The model under review builds one solid part; all positions refer to its coordinate system, in mm. Face numbers are marked on the shaded views. A direction names the side the tool comes from. Give positions to 0.01 mm unless a question says otherwise; leave off trailing zeros. Order: outer loops, then holes, each group sorted by start corner. A loop starts at its lowest first (then second) coordinate and runs counter-clockwise, first axis right, second up. Notation, with made-up numbers: (-21, -29.75) -> (-10, -29.75) arc R23 cw to (-10, 9.25) -> close; hole circle Ø9 at (-10.75, -9.75). An arc over 180 degrees is marked (long way). Use one line per item in the form item = value.
```python
from build123d import *

# Parameters (mm, degrees)
SKETCH1_W           = 25.4
SKETCH1_H           = 9.525
BOSS_EXTRUDE1_DEPTH = 12.7
SKETCH1_3_R         = 2.032
CUT_EXTRUDE1_DEPTH  = 4.7625
SKETCH3_R           = 2.032
CUT_EXTRUDE2_DEPTH  = 21.329919454
FILLET1_R           = 13.97
FILLET2_R           = 2.54
CHAMFER1_SIZE       = 0.635
CHAMFER2_SIZE       = 0.635
CHAMFER3_SIZE       = 0.635


with BuildPart() as part:
    # Sketch1 → Boss-Extrude1 (new body)
    with BuildSketch(Plane(origin=(0, 0, 0), x_dir=(1, 0, 0), z_dir=(0, 1, 0))):
        Rectangle(SKETCH1_W, SKETCH1_H)
    extrude(amount=BOSS_EXTRUDE1_DEPTH)

    # Sketch1<3> → Cut-Extrude1 (cut)
    with BuildSketch(Plane(origin=(0, 0, 0), x_dir=(1, 0, 0), z_dir=(0, 1, 0))):
        with Locations(Location((-6.35, 0, 0), (0, 0, 90))):
            Circle(SKETCH1_3_R)
        with Locations(Location((6.35, 0, 0), (0, 0, 90))):
            Circle(SKETCH1_3_R)
    extrude(amount=CUT_EXTRUDE1_DEPTH, mode=Mode.SUBTRACT)

    # Sketch3 → Cut-Extrude2 (cut, through all)
    with BuildSketch(Plane.XY.offset(4.7625)):
        Polygon((-12.7, 12.7), (-12.7, 6.35), (0, 12.7), align=None)
        Polygon((12.7, 12.7), (0, 12.7), (12.7, 6.35), align=None)
        with Locations((0, 7.62)):
            Circle(SKETCH3_R)
    extrude(amount=-CUT_EXTRUDE2_DEPTH, mode=Mode.SUBTRACT)

    # Fillet1
    fillet1_edges = [part.edges().sort_by_distance(p)[0] for p in [
        (0, 12.7, 0),
    ]]
    fillet(fillet1_edges, radius=FILLET1_R)

    # Fillet2
    fillet2_edges = [part.edges().sort_by_distance(p)[0] for p in [
        (-12.7, 6.35, 0),
        (12.7, 6.35, 0),
    ]]
    fillet(fillet2_edges, radius=FILLET2_R)

    # Chamfer1
    chamfer1_edges = [part.edges().sort_by_distance(p)[0] for p in [
        (-2.032, 7.62, -4.7625),
        (-2.032, 7.62, 4.7625),
    ]]
    chamfer(chamfer1_edges, length=CHAMFER1_SIZE)

    # Chamfer2
    chamfer2_edges = [part.edges().sort_by_distance(p)[0] for p in [
        (-6.35, 0, 2.032),
        (6.35, 0, 2.032),
    ]]
    chamfer(chamfer2_edges, length=CHAMFER2_SIZE)

    # Chamfer3
    chamfer3_edges = [part.edges().sort_by_distance(p)[0] for p in [
        (8.771748231, 8.314125885, 4.7625),
        (8.771748231, 8.314125885, -4.7625),
        (0, 0, -4.7625),
        (0, 11.051065177, 4.7625),
        (0, 11.051065177, -4.7625),
        (-12.7, 0, 0),
        (12.7, 2.390096834, -4.7625),
        (12.7, 2.390096834, 4.7625),
        (-8.771748231, 8.314125885, 4.7625),
        (-12.7, 2.390096834, 4.7625),
        (-12.320653053, 6.115550693, 4.7625),
        (0, 0, 4.7625),
        (12.320653053, 6.115550693, 4.7625),
        (-8.771748231, 8.314125885, -4.7625),
        (-12.7, 2.390096834, -4.7625),
        (-12.320653053, 6.115550693, -4.7625),
        (12.320653053, 6.115550693, -4.7625),
        (12.7, 0, 0),
    ]]
    chamfer(chamfer3_edges, length=CHAMFER3_SIZE)


solid = part.part
```
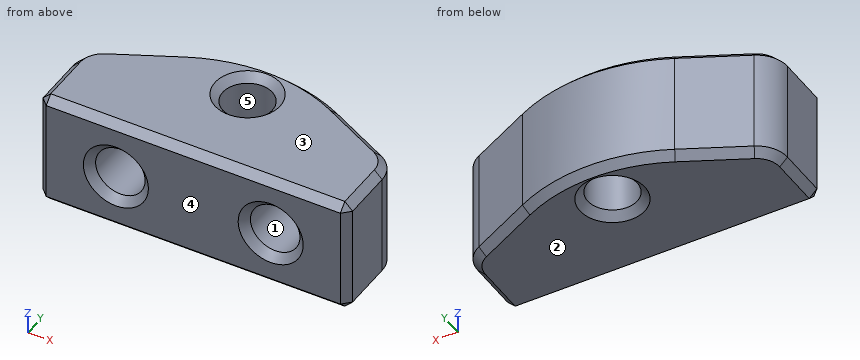
1. Add section C-C on y = 7.62. Give the boundary of the cut face in (x, z), then the cut area to 3 significant figures.
Values:
outline = (-10.16, -4.13) -> (-8.74, -4.76) -> (-2.67, -4.76) -> (-2.03, -4.13) -> (-2.03, 4.13) -> (-2.67, 4.76) -> (-8.74, 4.76) -> (-10.16, 4.13) -> close; (2.03, -4.13) -> (2.67, -4.76) -> (8.74, -4.76) -> (10.16, -4.13) -> (10.16, 4.13) -> (8.74, 4.76) -> (2.67, 4.76) -> (2.03, 4.13) -> close
area = 152 mm^2
2. Tool access review of the marked faces 1 and 2: name each direction out of +Z, -Z, +X, -X, +Y, -Y from which nothing blocks a thin tool from reaching the whole face with its end or side.
Values:
face_1 = -Y
face_2 = -Z, +X, -X, +Y, -Y
3. For L1, parallel to X at y = 1.9, z = 0; L2, parallel to Y at x = 0, z = -0.75; L3, parallel to X at y = 4.5, z = -1.25, list the stretches that pass through material, from the lowest coordinate up.
Values:
L1 = -12.7 to -8.38, -4.32 to 4.32, 8.38 to 12.7
L2 = 0 to 5.59, 9.65 to 11.05
L3 = -12.7 to -7.95, -4.75 to 4.75, 7.95 to 12.7
4. Add section B-B on y = 3. Count the separate pieces of the cut face and the enclosed holes in it, then the cut area to 3 significant figures.
Values:
separate_pieces = 1
enclosed_holes = 2
area = 215 mm^2
5. The part is to be moulded in two halves that separate along Y. For the marked faces 3, 4 and 5, say which applies: +Y half, -Y half, draft (parallel to the pull), parting line (faces both ways), or undercut.
Values:
face_3 = draft
face_4 = -Y half
face_5 = undercut
6. For pin 1 Ø4.5 at (x, z) = (6.35, 0) entering from -Y; pin 2 Ø4 at (x, z) = (-5.5, -0.5) entering from +Y; pin 3 Ø1.2 at (x, z) = (-6.5, 0) entering from -Y; pin 4 Ø3.5 at (x, y) = (0, 7.62) entering from -Z, all flat-tipped, find the tip position at first contact; note any pin that passes through.
Values:
pin_1 = 0.42
pin_2 = 10.61
pin_3 = 4.76
pin_4 = through
